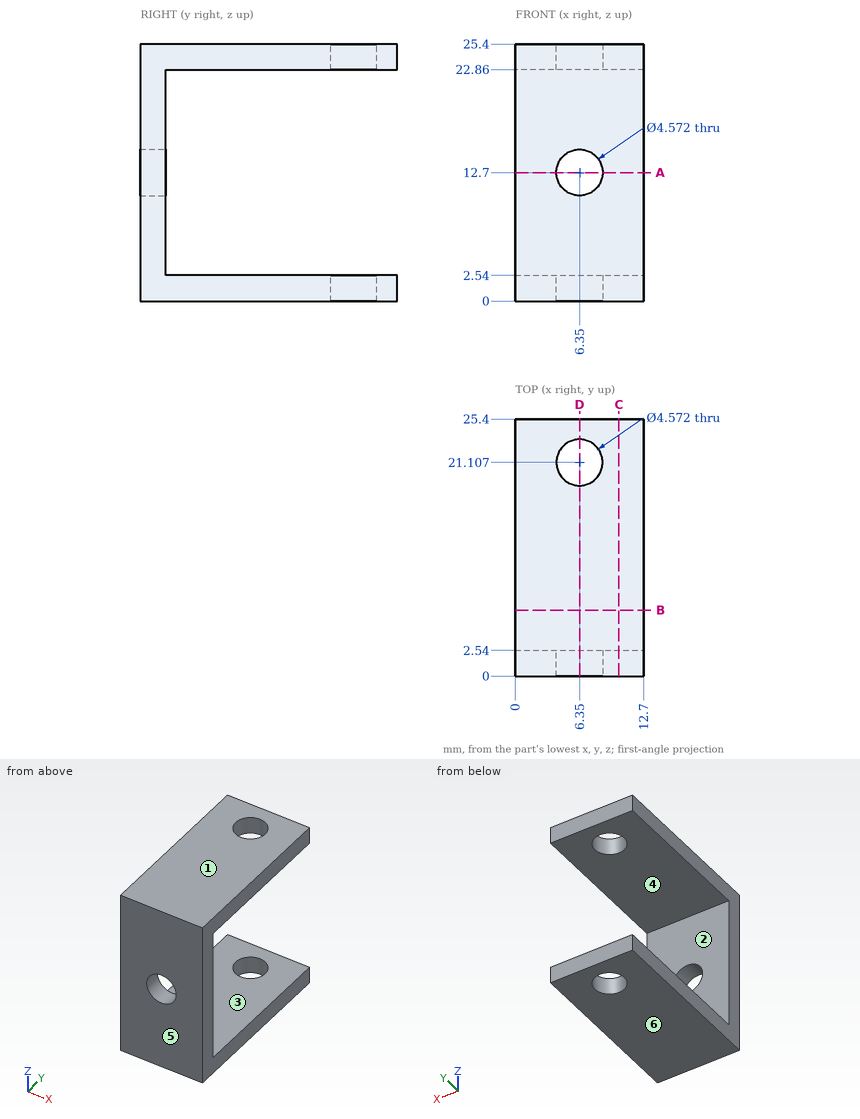
Can you work these out from the drawing? Everything is in mm from the part's minimum corner. A direction names the side the tool comes from. Round coordinates to 2 decimals unless told otherwise and drop trailing zeros. Write each loop counter-clockwise with the first axis right and the second up, starting at its lowest first coordinate (ties: lowest second). Pieces come first, ordered by that corner, then holes.
1. Will this pin go through, and if not, where does the flat tip stop? pin 1 Ø1 at (x, z) = (2, 21) entering from +Y.
2. For the marked faces 1 and 2, which set-ups out of +Z, -Z, +X, -X, +Y, -Y let a thin tool reach every point of the face, with its end or its side?
3. If we mould it in two halves opening along Z, with no side actions, what happens to the marked faces 3, 4, 5 and 6? For each: released by +Z, released by -Z, zero draft, split by the parting line, or undercut.
4. Suppose I cut it at B-B (y = 6.5). List the corners of the cut face in (x, z) for me.
5. Suppose I cut it at D-D (x = 6.35). List the corners of the cut face in (y, z) for me, and give its area (3 significant figures).
6. Suppose I cut it at A-A (z = 12.7). List the corners of the cut face in (x, y) for me.
7. I need wall thicknesses on L1, parallel to Z at x = 11.25, y = 8; L2, parallel to Z at x = 6.35, y = 1.75; L3, parallel to Y at x = 8, z = 18.5. Which ranges of each line are inside material? Lowest first, please.
8. Suppose I cut it at C-C (x = 10.25). List the corners of the cut face in (y, z) for me, and give its area (3 significant figures).
Answer sheet:
1. pin 1: stops at y = 2.54
2. face 1: +Z, +X, -X, +Y, -Y
2. face 2: +X, -X, +Y
3. face 3: undercut
3. face 4: undercut
3. face 5: zero draft
3. face 6: released by -Z
4. outline: (0, 0) - (12.7, 0) - (12.7, 2.54) - (0, 2.54) - close; (0, 22.86) - (12.7, 22.86) - (12.7, 25.4) - (0, 25.4) - close
5. outline: (0, 0) - (18.82, 0) - (18.82, 2.54) - (2.54, 2.54) - (2.54, 10.41) - (0, 10.41) - close; (0, 14.99) - (2.54, 14.99) - (2.54, 22.86) - (18.82, 22.86) - (18.82, 25.4) - (0, 25.4) - close; (23.39, 0) - (25.4, 0) - (25.4, 2.54) - (23.39, 2.54) - close; (23.39, 22.86) - (25.4, 22.86) - (25.4, 25.4) - (23.39, 25.4) - close
5. area: 146 mm2
6. outline: (0, 0) - (4.06, 0) - (4.06, 2.54) - (0, 2.54) - close; (8.64, 0) - (12.7, 0) - (12.7, 2.54) - (8.64, 2.54) - close
7. L1: z = 0 to 2.54, 22.86 to 25.4
7. L2: z = 0 to 10.41, 14.99 to 25.4
7. L3: y = 0 to 2.54
8. outline: (0, 0) - (25.4, 0) - (25.4, 2.54) - (2.54, 2.54) - (2.54, 22.86) - (25.4, 22.86) - (25.4, 25.4) - (0, 25.4) - close
8. area: 181 mm2
